from build123d import *

# Parameters (mm, degrees)
F0_W     = 200
F0_H     = 105
F1_DEPTH = 25
F2_T     = -2.5
F3_R     = 2.5
F4_DEPTH = 105


with BuildPart() as f1:
    # F0 (on Top) → F1 (new body)
    with BuildSketch(Plane.XY):
        Rectangle(F0_W, F0_H)
    extrude(amount=F1_DEPTH)

    # F2
    f2_openings = [f1.faces().sort_by_distance(p)[0] for p in [
        (0, 0, 25),
    ]]
    offset(amount=F2_T, openings=f2_openings)

    # F3 (on face) → F4 (cut, through all)
    with BuildSketch(Plane.XZ.offset(52.5)):
        with Locations((-91, 21)):
            Circle(F3_R)
        with Locations((-78, 21)):
            Circle(F3_R)
        with Locations((-65, 21)):
            Circle(F3_R)
        with Locations((-52, 21)):
            Circle(F3_R)
        with Locations((-39, 21)):
            Circle(F3_R)
        with Locations((-26, 21)):
            Circle(F3_R)
        with Locations((-13, 21)):
            Circle(F3_R)
        with Locations((0, 21)):
            Circle(F3_R)
        with Locations((13, 21)):
            Circle(F3_R)
        with Locations((26, 21)):
            Circle(F3_R)
        with Locations((39, 21)):
            Circle(F3_R)
        with Locations((52, 21)):
            Circle(F3_R)
        with Locations((65, 21)):
            Circle(F3_R)
        with Locations((78, 21)):
            Circle(F3_R)
        with Locations((91, 21)):
            Circle(F3_R)
    extrude(amount=-F4_DEPTH, mode=Mode.SUBTRACT)


solid = f1.part
For this review, take the finished solid that the model builds, in its own axes (mm). A direction names the side the tool comes from. Round coordinates to 2 decimals unless told otherwise and drop trailing zeros. Write each loop counter-clockwise with the first axis right and the second up, starting at its lowest first coordinate (ties: lowest second). Pieces come first, ordered by that corner, then holes. Notation, with made-up numbers: (-21.75, 7) -> (3.25, 7) arc R24 cw to (3.25, 37) -> close; hole circle Ø11 at (50, 56.5). An arc over 180 degrees is marked (long way). Put each result on its own line as item: value.
Q1. The part is to be moulded in two halves that separate along X. For faces 3 (the flat face through (-1, 52.5, 12)), 4 (the cylindrical face through (-13.33, 51.23, 23.48)), say which applies: released by +X, released by -X, zero draft, split by the parting line, or undercut.
Determined:
face 3: zero draft
face 4: undercut
Q2. Consider section A-A on z = 11. State the section outline as (x, y) points, and give its area (3 significant figures).
Determined:
outline: (-100, -52.5) -> (100, -52.5) -> (100, 52.5) -> (-100, 52.5) -> close; hole (-97.5, -50) -> (97.5, -50) -> (97.5, 50) -> (-97.5, 50) -> close
area: 1,500 mm^2
Q3. To check wall thickness, follow L1, parallel to X at y = 5, z = 7; L2, parallel to Z at x = -91, y = 51; L3, parallel to Y at x = 63.5, z = 15.5. State the ranges of each line that lie inside material, in increasing order. Write a range as [from, to].
Determined:
L1: x = [-100, -97.5], [97.5, 100]
L2: z = [0, 18.5], [23.5, 25]
L3: y = [-52.5, -50], [50, 52.5]
Q4. Clearance check with a flat-ended pin moving along its axis: pin 1 Ø3 at (x, y) = (-12, 27) entering from +Z. State where the tip first meets the part, or that it passes through.
Determined:
pin 1: stops at z = 2.5
Q5. Consider section B-B on x = 65. State the section outline as (y, z) points.
Determined:
outline: (-52.5, 0) -> (52.5, 0) -> (52.5, 18.5) -> (50, 18.5) -> (50, 2.5) -> (-50, 2.5) -> (-50, 18.5) -> (-52.5, 18.5) -> close; (-52.5, 23.5) -> (-50, 23.5) -> (-50, 25) -> (-52.5, 25) -> close; (50, 23.5) -> (52.5, 23.5) -> (52.5, 25) -> (50, 25) -> close
Q6. Consider section C-C on y = 2.5. State the section outline as (x, z) points.
Determined:
outline: (-100, 0) -> (100, 0) -> (100, 25) -> (97.5, 25) -> (97.5, 2.5) -> (-97.5, 2.5) -> (-97.5, 25) -> (-100, 25) -> close
Q7. Machinability: for faces 1 (the cylindrical face through (-63.66, -51.27, 23.11)), 2 (the flat face through (-1, 50, 14)), which of the approach directions +Z, -Z, +X, -X, +Y, -Y give a long, thin tool a straight path to every point of the face, cutting with its end or side? Answer none if there is none.
Determined:
face 1: +Y, -Y
face 2: +Z
